Source: CAD feature listing. Evaluate the final solid. Frame: model axes, mm. A direction names the side the tool comes from. Round coordinates to 2 decimals unless told otherwise and drop trailing zeros. Loops run counter-clockwise (first coordinate to the right, second up) from the corner with the lowest first, then second, coordinate; pieces in that order, holes last. Notation, with made-up numbers: M -38,59 L 21,59 A6 cw 21,67 Z; hole C -12,49 d4. An arc over 180 degrees is marked long. Answer as CSV lines item,"result". Start each with the question number.
```python
from build123d import *

# Parameters (mm, degrees)
CORTAR_EXTRUIR1_DEPTH = 6
CORTAR_EXTRUIR2_DEPTH = 4
MATRIZC1_COUNT        = 10
CROQUIS4_R            = 4
CORTAR_EXTRUIR3_DEPTH = 44.650429551


with BuildPart() as part:
    # Croquis1 → Revolución1 (revolve)
    with BuildSketch(Plane(origin=(0, 0, 0), x_dir=(0, 1, 0), z_dir=(0, 0, 1)), mode=Mode.PRIVATE) as revoluci_n1_sk:
        Polygon((0, 0), (19, 0), (19, 4), (13, 4), (13, 36), (10, 36), (10, 40.4), (0, 40.4), align=None)
    revolve(revoluci_n1_sk.sketch.rotate(Axis((0, 0, 0), (-1, 0, 0)), 90), axis=Axis((0, 0, 0), (-1, 0, 0)))

    # Croquis2 → Cortar-Extruir1 (cut)
    with BuildSketch(Plane.YZ):
        Polygon((2.485281374, -6), (6, -2.485281374), (6, 2.485281374), (2.485281374, 6), (-2.485281374, 6), (-6, 2.485281374), (-6, -2.485281374), (-2.485281374, -6), align=None)
    cortar_extruir1 = extrude(amount=-CORTAR_EXTRUIR1_DEPTH, mode=Mode.SUBTRACT)

    # Simetría1: Cortar-Extruir1 across plane
    add(cortar_extruir1.mirror(Plane(origin=(-20.2, 0, 0), x_dir=(0, 0, 1), z_dir=(1, 0, 0))), mode=Mode.SUBTRACT)

    # Croquis3 → Cortar-Extruir2 (cut)
    with BuildSketch(Plane.YZ):
        Polygon((2.25, 14.318019485), (2.25, 16.181980515), (0.931980515, 17.5), (-0.931980515, 17.5), (-2.25, 16.181980515), (-2.25, 14.318019485), (-0.931980515, 13), (0.931980515, 13), align=None)
    cortar_extruir2 = extrude(amount=-CORTAR_EXTRUIR2_DEPTH, mode=Mode.SUBTRACT)

    # MatrizC1: Cortar-Extruir2 ×10 about axis
    matrizc1_axis = Axis((0, 0, 0), (1, 0, 0))
    for i in range(1, MATRIZC1_COUNT):
        add(cortar_extruir2.rotate(matrizc1_axis, i * 360 / MATRIZC1_COUNT), mode=Mode.SUBTRACT)

    # Croquis4 → Cortar-Extruir3 (cut, through all)
    with BuildSketch(Plane.YZ.offset(-6)):
        with Locations(Location((0, 0, 0), (0, 0, 270))):
            Circle(CROQUIS4_R)
    extrude(amount=-CORTAR_EXTRUIR3_DEPTH, mode=Mode.SUBTRACT)


solid = part.part
```
1) Access query for faces 3 (the flat face through (-3, -6, 0)), 4 (the flat face through (-1.972, -10.776, -11.004)). Directions: +Z, -Z, +X, -X, +Y, -Y. A direction counts if a zero-diameter tool reaches every point of the face in a straight line with its end or side. Return the directions, or none.
2) Ray query, line 1 along Y through (x, z) = (-27.75, 0); line 2 along X through (y, z) = (-11.5, -5.5); line 3 along X through (y, z) = (-3.5, 17.5). Return the intervals inside material, ascending.
3) Section B-B, the plane x = -26. Return loops of the section in (y, z), and give its area (3 significant figures).
4) Mould query, pull axis Y, two halves, no side actions, for faces 1 (the flat face through (-6, -1.4, 4.1)), 2 (the flat face through (0, -4.5, -4.5)). Classes: pulls with the +Y half, pulls with the -Y half, needs draft (parallel to the pull), parting line crosses it, or undercut.
5) Section D-D, the plane x = -2.5. Give the number of separate pieces and of enclosed holes in the cut face, and give its area (3 significant figures).
6) Contact query for flat-ended pins moving along their axis: pin 1 Ø1.5 at (x, y) = (-20, -10) entering from -Z; pin 2 Ø0.6 at (x, y) = (-2.5, 0.5) entering from -Z; pin 3 Ø2 at (x, z) = (-3, 15) entering from -Y; pin 4 Ø7 at (y, z) = (0, 0) entering from +X. Output: stop coordinate, or through.
7) Section A-A, the plane z = 0. Return loops of the section in (x, y), and give its area (3 significant figures).
8) Section C-C, the plane y = 5. Return loops of the section in (x, z), and give its area (3 significant figures).
Findings below:
1,face 3,"+X"
1,face 4,"+X, -X"
2,line 1,"-13 to -4, 4 to 13"
2,line 2,"-36 to 0"
2,line 3,"-4 to 0"
3,outline,"C 0,0 d26; hole C 0,0 d8"
3,area,"481 mm²"
4,face 1,"undercut"
4,face 2,"needs draft"
5,separate pieces,"1"
5,enclosed holes,"11"
5,area,"847 mm²"
6,pin 1,"z = -9.13"
6,pin 2,"z = -19"
6,pin 3,"y = -12.85"
6,pin 4,"through"
7,outline,"M -40.4,-10 L -36,-10 L -36,-13 L -4,-13 L -4,-19 L 0,-19 L 0,-6 L -6,-6 L -6,-4 L -34.4,-4 L -34.4,-6 L -40.4,-6 Z; M -40.4,6 L -34.4,6 L -34.4,4 L -6,4 L -6,6 L 0,6 L 0,19 L -4,19 L -4,13 L -36,13 L -36,10 L -40.4,10 Z"
7,area,"701 mm²"
8,outline,"M -40.4,-8.66 L -36,-8.66 L -36,-12 L -4,-12 L -4,-18.33 L 0,-18.33 L 0,-3.49 L -6,-3.49 L -6,3.49 L 0,3.49 L 0,18.33 L -4,18.33 L -4,12 L -36,12 L -36,8.66 L -40.4,8.66 L -40.4,3.49 L -34.4,3.49 L -34.4,-3.49 L -40.4,-3.49 Z"
8,area,"907 mm²"
